Build history of the part. All positions in model axes, mm. Round coordinates to 2 decimals unless told otherwise and drop trailing zeros. Write each loop counter-clockwise with the first axis right and the second up, starting at its lowest first coordinate (ties: lowest second). Pieces come first, ordered by that corner, then holes. Notation, with made-up numbers: M 74.5,11.5 L 123.5,11.5 A7 ccw 123.5,20.5 Z; hole C -28.75,-10.75 d10. An arc over 180 degrees is marked long. Use a Markdown table: item, result.
from build123d import *

# Parameters (mm, degrees)
SKETCH_1_W          = 20
SKETCH_1_H          = 20
SKETCH_1_W_2        = 17
SKETCH_1_H_2        = 17
EXTRUDE_1_DEPTH     = 220
SKETCH_3_R          = 2
CUT_EXTRUDE_1_DEPTH = 23
SKETCH_4_R          = 3
CUT_EXTRUDE_2_DEPTH = 222.133443875


with BuildPart() as part:
    # 草图1 → 凸台-拉伸1 (new body)
    with BuildSketch(Plane.XY):
        Rectangle(SKETCH_1_W, SKETCH_1_H)
        Rectangle(SKETCH_1_W_2, SKETCH_1_H_2, mode=Mode.SUBTRACT)
    extrude(amount=EXTRUDE_1_DEPTH)

    # 草图3 → 切除-拉伸1 (cut)
    with BuildSketch(Plane.XZ.offset(10)):
        with Locations(Location((0, 20, 0), (0, 0, 270))):
            Circle(SKETCH_3_R)
        with Locations(Location((0, 5, 0), (0, 0, 270))):
            Circle(SKETCH_3_R)
    extrude(amount=-CUT_EXTRUDE_1_DEPTH, mode=Mode.SUBTRACT)

    # 草图4 → 切除-拉伸2 (cut, through all)
    with BuildSketch(Plane(origin=(0, 10, 0), x_dir=(1, 0, 0), z_dir=(0, 1, 0))):
        with Locations(Location((0, -55, 0), (0, 0, 270))):
            Circle(SKETCH_4_R)
    extrude(amount=-CUT_EXTRUDE_2_DEPTH, mode=Mode.SUBTRACT)


solid = part.part
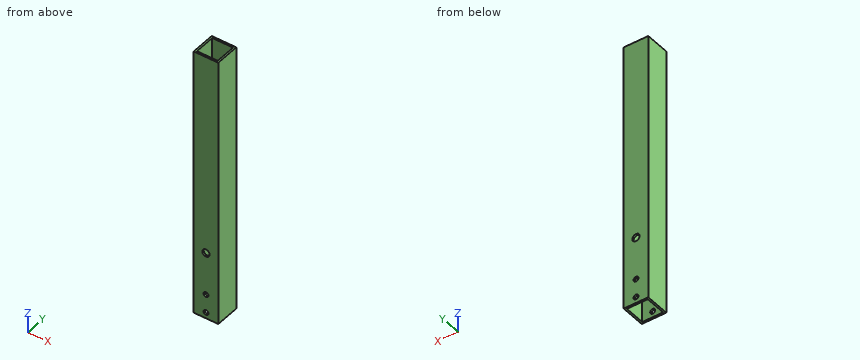
Q1. Drill centre lines: L1, parallel to X at y = -7.5, z = 60.5; L2, parallel to X at y = -9.45, z = 20. Where is each one in solid material? Low to high.
Response values:
| item | result |
|---|---|
| L1 | x = -10 to -8.5, 8.5 to 10 |
| L2 | x = -10 to -2, 2 to 10 |
Q2. Cut at A-A on z = 20. Give the cut face in (x, y).
Response values:
| item | result |
|---|---|
| outline | M -10,-10 L -2,-10 L -2,-8.5 L -8.5,-8.5 L -8.5,8.5 L -2,8.5 L -2,10 L -10,10 Z; M 2,-10 L 10,-10 L 10,10 L 2,10 L 2,8.5 L 8.5,8.5 L 8.5,-8.5 L 2,-8.5 Z |
Q3. Cut at B-B on x = -6.25. Give the cut face in (y, z).
Response values:
| item | result |
|---|---|
| outline | M -10,0 L -8.5,0 L -8.5,220 L -10,220 Z; M 8.5,0 L 10,0 L 10,220 L 8.5,220 Z |
Q4. Cut at D-D on z = 93. Give the cut face in (x, y), and give its area (3 significant figures).
Response values:
| item | result |
|---|---|
| outline | M -10,-10 L 10,-10 L 10,10 L -10,10 Z; hole M -8.5,-8.5 L 8.5,-8.5 L 8.5,8.5 L -8.5,8.5 Z |
| area | 111 mm2 |
